Source: CAD feature listing. Evaluate the final solid. Frame: model axes, mm. Round coordinates to 2 decimals unless told otherwise and drop trailing zeros. Write each loop counter-clockwise with the first axis right and the second up, starting at its lowest first coordinate (ties: lowest second). Pieces come first, ordered by that corner, then holes. Notation, with made-up numbers: (-19, -2) -> (-13, -2) arc R32 cw to (-13, 26) -> close; hole circle Ø1 at (41, 32). An arc over 180 degrees is marked (long way). Put each result on its own line as item: value.
```python
from build123d import *

# Parameters (mm, degrees)
BOSS_EXTRUDE1_DEPTH     = 1.5
CUT_EXTRUDE1_DEPTH      = 97.178219988
CUT_EXTRUDE1_DEPTH_BACK = 97.178219988
SKETCH3_W               = 30.375
SKETCH3_H               = 30.375
BOSS_EXTRUDE2_DEPTH     = 1.5


with BuildPart() as part:
    # Sketch1 → Boss-Extrude1 (new body)
    with BuildSketch(Plane.XY):
        Polygon((65, 38.88), (68, 38.88), (68, 12.76), (65, 12.76), (65, -13.06), (68, -13.06), (68, -39.18), (65, -39.18), (65, -65), (39.18, -65), (39.18, -68), (13.06, -68), (13.06, -65), (-12.76, -65), (-12.76, -68), (-38.88, -68), (-38.88, -65), (-64.7, -65), (-68, -65), (-68, -38.88), (-65, -38.88), (-65, -13.06), (-68, -13.06), (-68, 13.06), (-65, 13.06), (-65, 38.88), (-68, 38.88), (-68, 65), (-65, 65), (-65, 68), (-38.88, 68), (-38.88, 65), (-13.06, 65), (-13.06, 68), (13.06, 68), (13.06, 65), (38.88, 65), (38.88, 68), (65, 68), (65, 64.7), align=None)
    extrude(amount=BOSS_EXTRUDE1_DEPTH)

    # Sketch2 → Cut-Extrude1 (cut, two sides: drawn at the far end of the back side and taken through both)
    with BuildSketch(Plane.XY.offset(1.5).offset(-CUT_EXTRUDE1_DEPTH_BACK)):
        Polygon((63, -63), (37.18, -63), (37.18, -66), (15.06, -66), (15.06, -63), (-14.76, -63), (-14.76, -66), (-36.88, -66), (-36.88, -63), (-63, -63), (-66, -63), (-66, -40.88), (-63, -40.88), (-63, -11.06), (-66, -11.06), (-66, 11.06), (-63, 11.06), (-63, 40.88), (-66, 40.88), (-66, 63), (-63, 63), (-63, 66), (-40.88, 66), (-40.88, 63), (-11.06, 63), (-11.06, 66), (11.06, 66), (11.06, 63), (40.88, 63), (40.88, 66), (63, 66), (63, 63), (63, 36.88), (66, 36.88), (66, 14.76), (63, 14.76), (63, -15.06), (66, -15.06), (66, -37.18), (63, -37.18), align=None)
    extrude(amount=CUT_EXTRUDE1_DEPTH + CUT_EXTRUDE1_DEPTH_BACK, mode=Mode.SUBTRACT)

    # Sketch3 → Boss-Extrude2 (add, through all)
    with BuildSketch(Plane.XY.offset(1.5)):
        Polygon((0.75, -32.625), (31.125, -32.625), (31.125, -66), (32.625, -66), (32.625, -32.625), (66, -32.625), (66, -31.125), (32.625, -31.125), (32.625, -0.75), (63, -0.75), (63, 0.75), (32.625, 0.75), (32.625, 31.125), (66, 31.125), (66, 32.625), (32.625, 32.625), (32.625, 63), (31.125, 63), (31.125, 32.625), (0.75, 32.625), (0.75, 66), (-0.75, 66), (-0.75, 32.625), (-31.125, 32.625), (-31.125, 63), (-32.625, 63), (-32.625, 32.625), (-63, 32.625), (-63, 31.125), (-32.625, 31.125), (-32.625, 0.75), (-66, 0.75), (-66, -0.75), (-32.625, -0.75), (-32.625, -31.125), (-63, -31.125), (-63, -32.625), (-32.625, -32.625), (-32.625, -66), (-31.125, -66), (-31.125, -32.625), (-0.75, -32.625), (-0.75, -63), (0.75, -63), align=None)
        with Locations((-15.9375, -15.9375)):
            Rectangle(SKETCH3_W, SKETCH3_H, mode=Mode.SUBTRACT)
        with Locations((15.9375, -15.9375)):
            Rectangle(SKETCH3_W, SKETCH3_H, mode=Mode.SUBTRACT)
        with Locations((-15.9375, 15.9375)):
            Rectangle(SKETCH3_W, SKETCH3_H, mode=Mode.SUBTRACT)
        with Locations((15.9375, 15.9375)):
            Rectangle(SKETCH3_W, SKETCH3_H, mode=Mode.SUBTRACT)
    extrude(amount=-BOSS_EXTRUDE2_DEPTH)


solid = part.part
```
Q1. Cut plane C-C on z = 1. Give the number of separate pieces and of enclosed holes in the cut face, and give its area (3 significant figures).
Ans:
separate pieces: 1
enclosed holes: 16
area: 2,280 mm^2
Q2. Cut plane A-A on y = 27. Output: boundary loops of the cut face in (x, z) (3 decimals), and give its area (4 significant figures).
Ans:
outline: (-65, 0) -> (-63, 0) -> (-63, 1.5) -> (-65, 1.5) -> close; (-32.625, 0) -> (-31.125, 0) -> (-31.125, 1.5) -> (-32.625, 1.5) -> close; (-0.75, 0) -> (0.75, 0) -> (0.75, 1.5) -> (-0.75, 1.5) -> close; (31.125, 0) -> (32.625, 0) -> (32.625, 1.5) -> (31.125, 1.5) -> close; (66, 0) -> (68, 0) -> (68, 1.5) -> (66, 1.5) -> close
area: 12.75 mm^2
Q3. Pin query (flat end, axial travel): pin 1 (0.8 mm diameter, centred on x = 44, z = 0.5, fed in from -Y); pin 2 (0.8 mm diameter, centred on y = -48.5, z = 0.5, fed in from +X); pin 3 (0.8 mm diameter, centred on y = 23.5, z = 1, fed in from -X). Return the tip coordinate at first contact, or that it passes through.
Ans:
pin 1: stops at y = -65
pin 2: stops at x = 65
pin 3: stops at x = -65
Q4. Material intervals for line 1 (X direction, y = -22, z = 0.65) (3 decimals); line 2 (X direction, y = 11, z = 0.45) (3 decimals), sorted ascending. Write a range as [from, to].
Ans:
line 1: x = [-65, -63], [-32.625, -31.125], [-0.75, 0.75], [31.125, 32.625], [66, 68]
line 2: x = [-68, -66], [-32.625, -31.125], [-0.75, 0.75], [31.125, 32.625], [63, 65]
